from build123d import *

# Parameters (mm, degrees)
F1_DEPTH      = 150
F1_DEPTH_BACK = 150


with BuildPart() as f1:
    # F0 (on Right) → F1 (new body, two sides)
    with BuildSketch(Plane.YZ) as f1_sk:
        Polygon((0, 165.983751), (82.12112, 328.824738), (70.343, 319.571674), (-6.35, 167.494305), (-6.35, 53.473559), (20.889167, -21.175262), (28.124628, -22.479507), (2.355591, 48.140429), align=None)
    extrude(amount=F1_DEPTH)
    extrude(f1_sk.sketch, amount=-F1_DEPTH_BACK)


solid = f1.part
Work out the finished part from the listing and answer in its coordinate system (mm). Coordinates: 2 decimals unless noted, no trailing zeros. Write each loop counter-clockwise with the first axis right and the second up, starting at its lowest first coordinate (ties: lowest second). Pieces come first, ordered by that corner, then holes. Notation, with made-up numbers: M 0.25,60 L 30.25,60 A32 ccw 30.25,88 Z; hole C -5.75,-9 d5. An arc over 180 degrees is marked long. Write item = value, one per line.
1. The part is cut by section D-D (y = 32.5). Determine the outline of the cut face in (x, z), then the cut area to 3 significant figures.
Solution:
outline = M -150,230.43 L 150,230.43 L 150,244.53 L -150,244.53 Z
area = 4,230 mm2
2. The part is cut by section A-A (y = 11). Determine the outline of the cut face in (x, z).
Solution:
outline = M -150,5.93 L 150,5.93 L 150,24.45 L -150,24.45 Z; M -150,187.8 L 150,187.8 L 150,201.9 L -150,201.9 Z
3. Determine the mould class of faces 1 (the face through (2.1, 40.486, 246.264)), 2 (the face through (2.1, 7.08, 16.67)), 3 (the face through (2.1, 15.42, 12.34)), 4 (the face through (150, -2, 141)) for opening direction Z: released by +Z, released by -Z, zero draft, split by the parting line, or undercut.
Solution:
face_1 = undercut
face_2 = released by -Z
face_3 = undercut
face_4 = zero draft
4. The part is cut by section C-C (z = 211). Determine the outline of the cut face in (x, y), then the cut area to 3 significant figures.
Solution:
outline = M -150,15.59 L 150,15.59 L 150,22.7 L -150,22.7 Z
area = 2,130 mm2
5. Flat-ended cylindrical pins translate along their axes: pin 1 (5 mm diameter, centred on x = 66.5, y = 65, fed in from +Z); pin 2 (6 mm diameter, centred on x = 107, z = 275, fed in from -Y); pin 3 (3 mm diameter, centred on x = -92, y = 19.5, fed in from +Z). Find the tip coordinate at first contact, or state that the pin passes through.
Solution:
pin_1 = 313.93
pin_2 = 46.35
pin_3 = 221.73
6. The part is cut by section B-B (x = 78). Determine the outline of the cut face in (y, z), then the cut area to 3 significant figures.
Solution:
outline = M -6.35,53.47 L 20.89,-21.18 L 28.12,-22.48 L 2.36,48.14 L 0,165.98 L 82.12,328.82 L 70.34,319.57 L -6.35,167.49 Z
area = 2,480 mm2
7. Straight lines are drawn through the part: line 1 (Y direction, x = 127, z = 33.5); line 2 (Y direction, x = 69, z = 271.5); line 3 (Z direction, x = -77.5, y = 41). For each, find the intervals that lie inside material, in ascending order. Write a range as from..to.
Solution:
line_1 = 0.94..7.7
line_2 = 46.1..53.21
line_3 = 247.28..261.39
